Autodesk Inventor part; units mm, degrees
ref_plane "YZ Plane" through (0, 0, 0) normal (1, 0, 0) x (0, 1, 0)
ref_plane "XZ Plane" through (0, 0, 0) normal (0, 1, 0) x (-1, 0, 0)
ref_plane "XY Plane" through (0, 0, 0) normal (0, 0, 1) x (1, 0, 0)
sketch "Skizze1" plane through (0, 0, 0) normal (1, 0, 0) x (0, 1, 0)
  circle A0 centre (0, 0) radius 6
  circle A1 centre (0, 0) radius 3
  dimension "d0" = 12
  dimension "d1" = 6
extrude "Extrusion1" add sketch "Skizze1" along normal blind 30.55
sketch "Skizze2" plane through (0, 0, 0) normal (0, 1, 0) x (-1, 0, 0)
  line L0 (-30.55, 6) -> (-30.55, -6) construction
  line L1 (-30.55, 6) -> (-30.55, -6) construction
  line L2 (-30.55, 6) -> (-26.55, 6)
  line L3 (0, 6) -> (-30.55, 6)
  line L4 (-30.55, 6) -> (-30.55, 6.1)
  line L5 (-30.55, 6) -> (-26.7263, 7)
  line L6 (-26.7263, 7) -> (-26.55, 6)
  point P0 (0, 0)
  dimension "d4" = 4
  dimension "d5" = 0.1
  dimension "d6" = 80
  dimension "d7" = 1
coil "Spirale1" sketch "Skizze2" operation add axis through (-10, 0, 0) along (-1, 0, 0) pitch 7 turns 2.7 hand right
mirror "Spiegeln1" about plane through (0, 0, 0) normal (1, 0, 0) of "Extrusion1", "Spirale1"
sketch "Skizze3" plane through (30.55, 0, 0) normal (1, 0, 0) x (0, 0, -1)
  circle A0 centre (0, 0) radius 5
  dimension "d16" = 10
extrude "Extrusion2" cut sketch "Skizze3" against normal blind 4
properties part number "Dribblerschnecke"
Geometry check sheet. Reference: the model listing, model coordinates, mm. A direction names the side the tool comes from. Coordinates: 2 decimals unless noted, no trailing zeros. Order: outer loops, then holes, each group sorted by start corner. A loop starts at its lowest first (then second) coordinate and runs counter-clockwise, first axis right, second up. Notation, with made-up numbers: M -0.5,31 L 18.5,31 A10 cw 18.5,35 Z; hole C 15,-1.5 d5. An arc over 180 degrees is marked long. One line per question, with ' | ' between items. Start each with the question number.
Item 1: Material ranges on L1, parallel to Z at x = 9, y = 0; L2, parallel to Y at x = 29.1, z = 0, recorded low to high. Write a range as [from, to].
Item 2: Set-up check for faces 1 (the flat face through (26.55, 0.1, -3.3)), 2 (the flat face through (28.1, 0, 6.4)), 3 (the cylindrical face through (-2, -3, 0)), 4 (the flat face through (-27.7, 0, 6.4)): record each of +Z, -Z, +X, -X, +Y, -Y from which the full face is reachable in a straight line by a thin tool's end or side.
Item 3: Gauge pin test, flat ends, axial feed: pin 1 (5 mm diameter, centred on x = -4.5, z = 0, fed in from -Y); pin 2 (5 mm diameter, centred on x = 17, z = 3.5, fed in from +Y); pin 3 (1 mm diameter, centred on x = -12.5, y = 3, fed in from -Z). Record the tip position at first contact, or that the pin passes through.
Item 4: Cross-section at A-A on x = -7. Enter the section's corners in (y, z).
Item 5: Draft check along Z on faces 5 (the flat face through (30.55, -4, 4)), 6 (the cylindrical face through (28.58, -4.88, 1.08)). Enter one of: pulls with the +Z half, pulls with the -Z half, needs draft (parallel to the pull), parting line crosses it, or undercut.
Findings:
1) L1: z = [-6, -3], [3, 6] | L2: y = [-6, -5], [5, 6]
2) face 1: +X | face 2: +Z, +X, -Y | face 3: +X, -X | face 4: +Z, -X, -Y
3) pin 1: stops at y = -6 | pin 2: stops at y = 6.88 | pin 3: stops at z = -5.79
4) outline: C 0,0 d12; hole C 0,0 d6
5) face 5: needs draft | face 6: undercut
